Geometry check sheet. Reference: the model listing, model coordinates, mm. A direction names the side the tool comes from. Coordinates: 2 decimals unless noted, no trailing zeros. Loops run counter-clockwise (first coordinate to the right, second up) from the corner with the lowest first, then second, coordinate; pieces in that order, holes last.
from build123d import *

# Parameters (mm, degrees)
F1_DEPTH = 25
F2_DEPTH = 25


# Not quite as in the source:
# - a feature of the source that left no trace in its solid (it failed there, or was rolled back) is left out


with BuildPart() as f1:
    # F0 (on Front) → F1 (new body)
    with BuildSketch(Plane.XZ):
        with BuildLine():
            Line((20, 30), (0, 0))
            Line((0, 0), (-20, 30))
            Line((-20, 30), (-30, 30))
            Line((-30, 30), (-44.90711985, 13.3333333333))
            ThreePointArc((-44.90711985, 13.3333333333), (-50, 0), (-44.90711985, -13.3333333333))
            Line((-44.90711985, -13.3333333333), (-30, -30))
            Line((-30, -30), (-17.3205080757, -30))
            ThreePointArc((-17.3205080757, -30), (0, -20), (17.3205080757, -30))
            Line((17.3205080757, -30), (30, -30))
            Line((30, -30), (30, 30))
            Line((30, 30), (20, 30))
        make_face()
    extrude(amount=F1_DEPTH)

    # F2 (add): a face of the model
    f2_faces = [f1.faces().sort_by_distance(p)[0] for p in [
        (-8.0009938, -25, -1.613641283),
    ]]
    extrude(f2_faces, amount=F2_DEPTH)


solid = f1.part
1) Mould release check, pull along X, two halves, no side actions. Record for faces 1 (the flat face through (-37.35, -24.65, 21.78)), 2 (the cylindrical face through (0, -25, -20)), 3 (the flat face through (10, -25, 15)), 4 (the flat face through (25, -25, 30)): +X half, -X half, draft (parallel to the pull), parting line (faces both ways), or undercut.
Data:
face 1: -X half
face 2: undercut
face 3: undercut
face 4: draft
2) Access from +Z, -Z, +X, -X, +Y, -Y to the whole of each face (thin tool, end or side, straight path). Record for faces 5 (the cylindrical face through (-50, -25, 0)), 6 (the flat face through (-10, -25, 15)).
Data:
face 5: -X, +Y, -Y
face 6: +Z, +Y, -Y
3) Section check B-B on z = 22.5. Record the cut outline in (x, y).
Data:
outline: (-36.71, -50) - (-15, -50) - (-15, 0) - (-36.71, 0) - close; (15, -50) - (30, -50) - (30, 0) - (15, 0) - close
4) Section check D-D on x = -16. Record the cut outline in (y, z).
Data:
outline: (-50, -28) - (0, -28) - (0, 24) - (-50, 24) - close
5) Section check A-A on y = -46. Record the cut outline in (x, z).
Data:
outline: (-44.91, -13.33) - (-30, -30) - (-17.32, -30) arc R20 cw to (17.32, -30) - (30, -30) - (30, 30) - (20, 30) - (0, 0) - (-20, 30) - (-30, 30) - (-44.91, 13.33) arc R20 ccw to start
6) Section check C-C on z = -12. Record the cut outline in (x, y), and give its area (3 significant figures).
Data:
outline: (-46, -50) - (30, -50) - (30, 0) - (-46, 0) - close
area: 3,800 mm2
7) Material ranges on probe 1 along X at (y, z) = (-32.5, 1); probe 2 along X at (y, z) = (-20, -22); probe 3 along Z at (x, y) = (-14, -6.5), recorded low to high.
Data:
probe 1: x = -49.97 to -0.67, 0.67 to 30
probe 2: x = -37.16 to -8.72, 8.72 to 30
probe 3: z = -25.72 to 21
8) Depth check by flat-ended pin: pin 1 (2 mm diameter, centred on x = -36.5, y = -39, fed in from +Z); pin 2 (10 mm diameter, centred on y = -19, z = 2, fed in from -X); pin 3 (3 mm diameter, centred on y = -34, z = -16, fed in from -X); pin 4 (1.5 mm diameter, centred on x = -20.5, z = -5.5, fed in from +Y). Enter the tip coordinate at first touch or a pass-through.
Data:
pin 1: stops at z = 23.85
pin 2: stops at x = -50
pin 3: stops at x = -43.86
pin 4: stops at y = 0
